Source: CAD feature listing. Evaluate the final solid. Frame: model axes, mm. A direction names the side the tool comes from. Give positions to 0.01 mm unless a question says otherwise; leave off trailing zeros. Loops run counter-clockwise (first coordinate to the right, second up) from the corner with the lowest first, then second, coordinate; pieces in that order, holes last. Notation, with made-up numbers: (28.25, 43) - (40.25, 43) arc R14 cw to (40.25, 49) - close; hole circle Ø5 at (14, -29.75). An arc over 180 degrees is marked (long way). Put each result on its own line as item: value.
```python
from build123d import *

# Parameters (mm, degrees)
F0_R     = 7.9375
F1_DEPTH = 6.35
F0_R_2   = 9.19734
F2_DEPTH = 3.175
F3_R     = 2.54


with BuildPart() as f1:
    # F0 (on Top) → F1 (new body)
    with BuildSketch(Plane.XY):
        Circle(F0_R)
    extrude(amount=F1_DEPTH)

    # F0 (on Top) → F2 (join)
    with BuildSketch(Plane.XY):
        Circle(F0_R_2)
        Circle(F0_R, mode=Mode.SUBTRACT)
    extrude(amount=F2_DEPTH)

    # F3
    f3_edges = [f1.edges().sort_by_distance(p)[0] for p in [
        (-9.19734, 0, 0),
    ]]
    fillet(f3_edges, radius=F3_R)


solid = f1.part
```
1) Section query C-C, the plane z = 5.75. Output: boundary loops of the cut face in (x, y) (1 decimal).
Check result:
outline: circle Ø15.9 at (0, 0)
2) Access query for faces 1 (the cylindrical face through (-1.72, -7.75, 4.74)), 2 (the flat face through (0, 0, 6.35)). Directions: +Z, -Z, +X, -X, +Y, -Y. A direction counts if a zero-diameter tool reaches every point of the face in a straight line with its end or side. Return the directions, or none.
Check result:
face 1: +Z
face 2: +Z, +X, -X, +Y, -Y
3) Section query D-D, the plane z = 1.75. Output: boundary loops of the cut face in (x, y), plus the area to 3 significant figures.
Check result:
outline: circle Ø18.14 at (0, 0)
area: 259 mm²
4) Pin query (flat end, axial travel): P1, Ø2, axis at x = -7, z = 5.5, coming from the +Y side; P2, Ø1, axis at y = 5, z = 4.5, coming from the +X side. Return the tip coordinate at first contact, or that it passes through.
Check result:
P1: y = 5.2
P2: x = 6.54
5) Material intervals for line 1 along X through (y, z) = (0.25, 2.5); line 2 along Y through (x, z) = (5.5, 4), sorted ascending. Write a range as [from, to].
Check result:
line 1: [-9.19, 9.19]
line 2: [-5.72, 5.72]
